```python
from build123d import *

# Parameters (mm, degrees)
F1_DEPTH = 6.35
F2_R     = 1.5875
F3_DEPTH = 3.175


# Not quite as in the source:
# - a feature of the source that left no trace in its solid (it failed there, or was rolled back) is left out


with BuildPart() as f1:
    # F0 (on Front) → F1 (new body)
    with BuildSketch(Plane.XZ):
        Polygon((-57.817878572, 25.3623127937), (-65.437878572, 6.3123127937), (-19.717878572, 6.3123127937), (-27.337878572, 25.3623127937), (-42.577878572, 25.3623127937), align=None)
    extrude(amount=F1_DEPTH)

    # F2 (on face) → F3 (join)
    with BuildSketch(Plane.XZ.offset(6.35)):
        with Locations((-58.452878572, 9.4873127937)):
            Circle(F2_R)
        with Locations((-26.702878572, 9.4873127937)):
            Circle(F2_R)
        with Locations((-42.577878572, 22.1873127937)):
            Circle(F2_R)
    extrude(amount=F3_DEPTH)


solid = f1.part
```
Geometry check sheet. Reference: the model listing, model coordinates, mm. A direction names the side the tool comes from. Coordinates: 2 decimals unless noted, no trailing zeros. Order: outer loops, then holes, each group sorted by start corner. A loop starts at its lowest first (then second) coordinate and runs counter-clockwise, first axis right, second up. Notation, with made-up numbers: (39.5, 42.5) - (71.5, 42.5) arc R16 ccw to (71.5, 61.5) - close; hole circle Ø11 at (-39, -29). An arc over 180 degrees is marked (long way). Answer in a Markdown table with one row per item. Add a question column.
1. Section check C-C (x = -53). Enter the section's corners in (y, z).
2. Gauge pin test, flat ends, axial feed: pin 1 Ø1 at (x, z) = (-31.5, 10) entering from -Y; pin 2 Ø1 at (y, z) = (-8, 9.5) entering from +X; pin 3 Ø3 at (y, z) = (-8, 23.5) entering from -X. Record the tip position at first contact, or that the pin passes through.
3. Access from +Z, -Z, +X, -X, +Y, -Y to the whole of each face (thin tool, end or side, straight path). Record for faces 4 (the face through (-43, -6.35, 16)), 5 (the face through (-43, -3, 6.312)).
4. Section check B-B (y = -7.5). Enter the section's corners in (x, z) (1 decimal).
5. Material ranges on L1, parallel to Y at x = -57.5, z = 16.5; L2, parallel to Z at x = -58.5, y = -6.5; L3, parallel to X at y = -4.5, z = 8.75, recorded low to high. Write a range as [from, to].
6. Draft check along X on faces 1 (the face through (-61.575, -3.131, 15.971)), 2 (the face through (-58, -9.525, 10)), 3 (the face through (-56.939, -7.915, 9.964)). Enter one of: +X half, -X half, draft (parallel to the pull), parting line (faces both ways), or undercut.
7. Section check D-D (y = -5.5). Enter the section's corners in (x, z), plus the area to 3 significant figures.
8. Section check A-A (z = 10.25). Enter the section's corners in (x, y) (3 decimals).
Data:
| question | item | result |
|---|---|---|
| 1 | outline | (-6.35, 6.31) - (0, 6.31) - (0, 25.36) - (-6.35, 25.36) - close |
| 2 | pin 1 | stops at y = -6.35 |
| 2 | pin 2 | stops at x = -25.12 |
| 2 | pin 3 | stops at x = -44.17 |
| 3 | face 4 | -Y |
| 3 | face 5 | -Z, +X, -X, +Y, -Y |
| 4 | outline | circle Ø3.2 at (-58.5, 9.5); circle Ø3.2 at (-42.6, 22.2); circle Ø3.2 at (-26.7, 9.5) |
| 5 | L1 | y = [-6.35, 0] |
| 5 | L2 | z = [7.9, 11.07] |
| 5 | L3 | x = [-64.46, -20.69] |
| 6 | face 1 | -X half |
| 6 | face 2 | draft |
| 6 | face 3 | undercut |
| 7 | outline | (-65.44, 6.31) - (-19.72, 6.31) - (-27.34, 25.36) - (-57.82, 25.36) - close |
| 7 | area | 726 mm² |
| 8 | outline | (-63.863, -6.35) - (-59.845, -6.35) - (-59.845, -9.525) - (-57.061, -9.525) - (-57.061, -6.35) - (-28.095, -6.35) - (-28.095, -9.525) - (-25.311, -9.525) - (-25.311, -6.35) - (-21.293, -6.35) - (-21.293, 0) - (-63.863, 0) - close |
